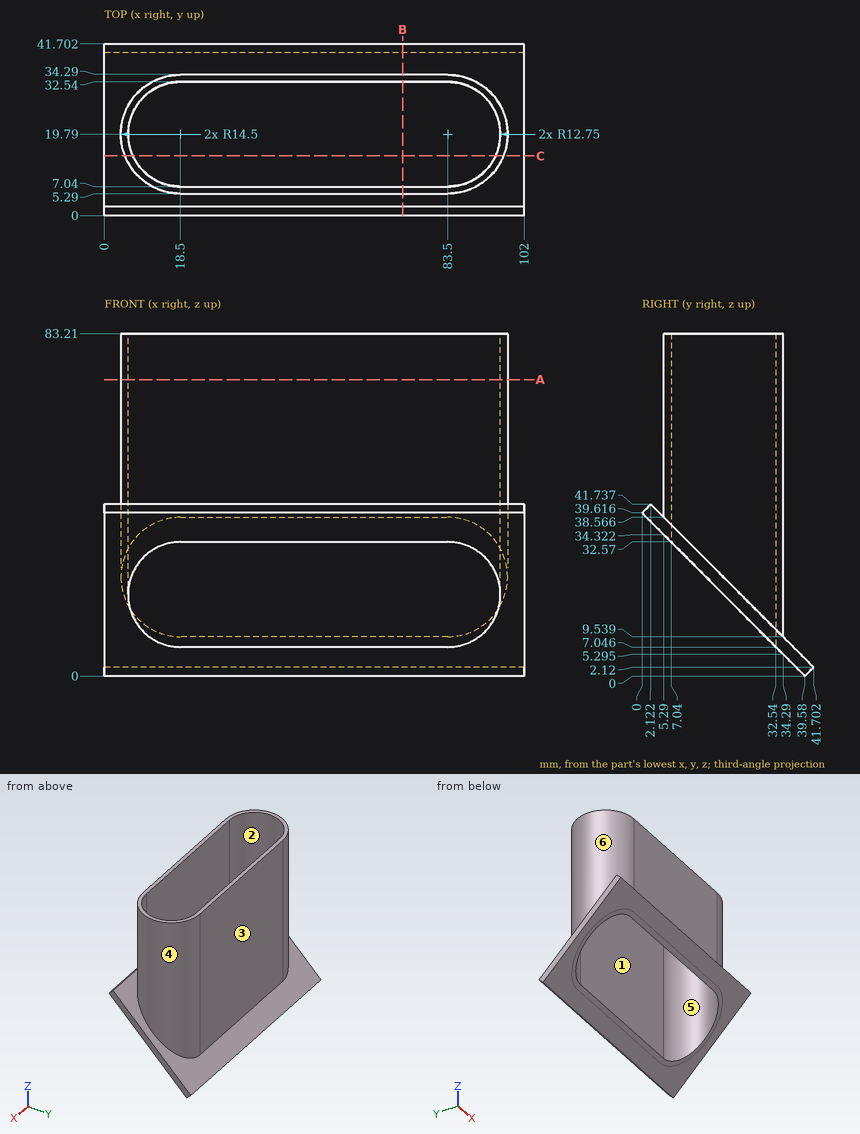
Here's the drawing with two shaded views (mm, measured from the low corner). I have some questions. A direction names the side the tool comes from. Give positions to 0.01 mm unless a question says otherwise; leave off trailing zeros. Order: outer loops, then holes, each group sorted by start corner. A loop starts at its lowest first (then second) coordinate and runs counter-clockwise, first axis right, second up. Notation, with made-up numbers: M -30.75,0 L 24.25,0 A31 cw 24.25,31 Z; hole C 1,62 d3. An arc over 180 degrees is marked long. One line per item, written item: value.
1) Please list where these lines run through material, in increasing order: line 1 along Y through (x, z) = (19, 60.5); line 2 along Y through (x, z) = (14, 51) (1 decimal); line 3 along X through (y, z) = (23.5, 71.5).
Answer sheet:
line 1: y = 5.29 to 7.04, 32.54 to 34.29
line 2: y = 6 to 7.9, 31.7 to 33.6
line 3: x = 4.48 to 6.3, 95.7 to 97.52
2) We'd pull the mould along Y, two halves only. Please class the marked faces 1, 2 and 3: released by +Y, released by -Y, zero draft, split by the parting line, or undercut.
Answer sheet:
face 1: undercut
face 2: undercut
face 3: released by +Y
3) I want a section at C-C, the plane y = 14.5. List the corners of the cut face in (x, z) for me.
Answer sheet:
outline: M 0,25.1 L 6.9,25.1 L 6.9,83.21 L 5,83.21 L 5,29.35 L 0,29.35 Z; M 95.1,25.1 L 102,25.1 L 102,29.35 L 97,29.35 L 97,83.21 L 95.1,83.21 Z
4) I want a section at B-B, the plane x = 72.5. List the corners of the cut face in (y, z) for me (1 decimal), plus the area to 3 significant figures.
Answer sheet:
outline: M 0,39.6 L 7,32.6 L 7,83.2 L 5.3,83.2 L 5.3,38.6 L 2.1,41.7 Z; M 32.5,7 L 39.6,0 L 41.7,2.1 L 34.3,9.5 L 34.3,83.2 L 32.5,83.2 Z
area: 267 mm^2
5) For P1, Ø10, axis at y = 4, z = 49.5, coming from the -X side (1 decimal); P2, Ø13.5, axis at x = 50, z = 52.5, coming from the -Y side; P3, Ø10, axis at x = 12.5, y = 13.5, coming from the -Z side (1 decimal), each with a flat end and sliding along its axis, tell me the tip position at first contact or that it passes through.
Answer sheet:
P1: stops at x = 8.8
P2: stops at y = 5.29
P3: stops at z = 26.3
6) I want a section at A-A, the plane z = 72. List the corners of the cut face in (x, y) for me.
Answer sheet:
outline: M 18.5,5.29 L 83.5,5.29 A14.5 ccw 83.5,34.29 L 18.5,34.29 A14.5 ccw Z; hole M 18.5,7.04 L 83.5,7.04 A12.75 ccw 83.5,32.54 L 18.5,32.54 A12.75 ccw Z
7) On a 3-axis mill with a long thin cutter (end or side, diameter ignored), from which of +Z, -Z, +X, -X, +Y, -Y can I reach the whole of each face in a straight line? I mean the marked faces 4, 5 and 6. Say none if no direction works.
Answer sheet:
face 4: +Z, +X
face 5: +Z, -Z
face 6: +Z, -X
